The model under review builds one solid part; all positions refer to its coordinate system, in mm. Face numbers are marked on the shaded views. A direction names the side the tool comes from. Coordinates: 2 decimals unless noted, no trailing zeros. Write each loop counter-clockwise with the first axis right and the second up, starting at its lowest first coordinate (ties: lowest second). Pieces come first, ordered by that corner, then holes. Notation, with made-up numbers: (75, 86.25) - (85, 86.25) arc R29 cw to (85, 125.25) - close; hole circle Ø6 at (-25, 50). An arc over 180 degrees is marked (long way). Put each result on its own line as item: value.
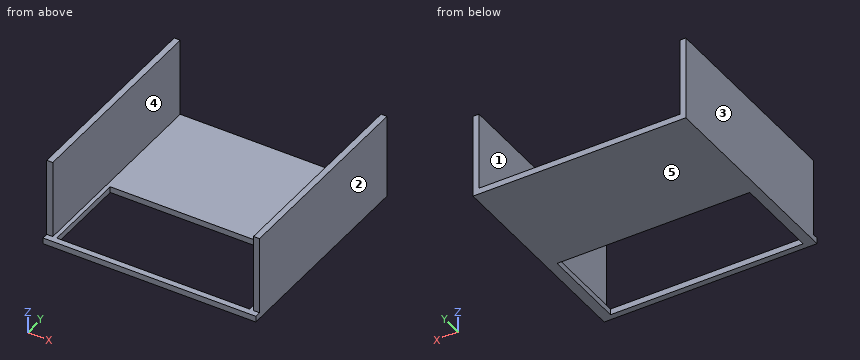
from build123d import *

# Parameters (mm, degrees)
SKETCH1_W                = 100
SKETCH1_H                = 77.5
BOSS_EXTRUDE1_DEPTH      = 3
BOSS_EXTRUDE2_DEPTH      = 102.5
BOSS_EXTRUDE2_DEPTH_BACK = 3
SKETCH2_W                = 106
SKETCH2_H                = 83.5
SKETCH2_W_2              = 100
SKETCH2_H_2              = 77.5
SKETCH3_W                = 106
SKETCH3_H                = 105.5
CUT_EXTRUDE1_DEPTH       = 41.5
CUT_EXTRUDE3_REACH       = 127.313
SKETCH6_W                = 96
SKETCH6_H                = 43
SKETCH7_W                = 106
SKETCH7_H                = 3
CUT_EXTRUDE4_DEPTH       = 39


with BuildPart() as part:
    # Sketch1 → Boss-Extrude1 (new body)
    with BuildSketch(Plane(origin=(0, 0, 0), x_dir=(1, 0, 0), z_dir=(0, 1, 0))):
        Rectangle(SKETCH1_W, SKETCH1_H)
    extrude(amount=BOSS_EXTRUDE1_DEPTH)

    # Sketch2 → Boss-Extrude2 (add, two sides: drawn at the far end of the back side and taken through both)
    with BuildSketch(Plane(origin=(0, 3, 0), x_dir=(1, 0, 0), z_dir=(0, 1, 0)).offset(-BOSS_EXTRUDE2_DEPTH_BACK)):
        Rectangle(SKETCH2_W, SKETCH2_H)
        Rectangle(SKETCH2_W_2, SKETCH2_H_2, mode=Mode.SUBTRACT)
    extrude(amount=BOSS_EXTRUDE2_DEPTH + BOSS_EXTRUDE2_DEPTH_BACK)

    # Sketch3 → Cut-Extrude1 (cut)
    with BuildSketch(Plane(origin=(0, 0, 41.75), x_dir=(-1, 0, 0), z_dir=(0, 0, -1))):
        with Locations((0, 52.75)):
            Rectangle(SKETCH3_W, SKETCH3_H)
    extrude(amount=CUT_EXTRUDE1_DEPTH, mode=Mode.SUBTRACT)

    # Sketch6 → Cut-Extrude3 (cut, up to next)
    with BuildSketch(Plane(origin=(0, 0, -41.75), x_dir=(-1, 0, 0), z_dir=(0, 0, -1)), mode=Mode.PRIVATE) as cut_extrude3_sk1:
        with Locations((0, 24.5)):
            Rectangle(SKETCH6_W, SKETCH6_H)
    cut_extrude3_tool1 = extrude(cut_extrude3_sk1.sketch, amount=-CUT_EXTRUDE3_REACH, mode=Mode.PRIVATE) & part.part
    add(cut_extrude3_tool1.solids().sort_by_distance((0, 24.5, -41.75))[0], mode=Mode.SUBTRACT)

    # Sketch7 → Cut-Extrude4 (cut)
    with BuildSketch(Plane.XY.offset(0.25)):
        with Locations((0, 1.5)):
            Rectangle(SKETCH7_W, SKETCH7_H)
    extrude(amount=-CUT_EXTRUDE4_DEPTH, mode=Mode.SUBTRACT)


solid = part.part
1. Consider section D-D on y = 68. State the section outline as (x, z) points, plus the area to 3 significant figures.
Determined:
outline: (-53, -41.75) - (53, -41.75) - (53, 0.25) - (50, 0.25) - (50, -38.75) - (-50, -38.75) - (-50, 0.25) - (-53, 0.25) - close
area: 552 mm^2
2. Consider section A-A on x = 44. State the section outline as (y, z) points, plus the area to 4 significant figures.
Determined:
outline: (0, -41.75) - (3, -41.75) - (3, -38.75) - (0, -38.75) - close; (46, -41.75) - (105.5, -41.75) - (105.5, -38.75) - (46, -38.75) - close
area: 187.5 mm^2
3. Consider section C-C on y = 15. State the section outline as (x, z) points, plus the area to 3 significant figures.
Determined:
outline: (-53, -41.75) - (-48, -41.75) - (-48, -38.75) - (-50, -38.75) - (-50, 0.25) - (-53, 0.25) - close; (48, -41.75) - (53, -41.75) - (53, 0.25) - (50, 0.25) - (50, -38.75) - (48, -38.75) - close
area: 264 mm^2
4. To check wall thickness, follow probe 1 along X at (y, z) = (66, -23); probe 2 along Y at (x, z) = (9, -39.5); probe 3 along X at (y, z) = (40.5, -40). State the ranges of each line that lie inside material, in increasing order.
Determined:
probe 1: x = -53 to -50, 50 to 53
probe 2: y = 0 to 3, 46 to 105.5
probe 3: x = -53 to -48, 48 to 53
5. Machinability: for the marked faces 4 and 5, which of the approach directions +Z, -Z, +X, -X, +Y, -Y give a long, thin tool a straight path to every point of the face, cutting with its end or side? Answer none if there is none.
Determined:
face 4: +Z, +Y, -Y
face 5: -Z, +X, -X, +Y, -Y
6. The part is to be moulded in two halves that separate along X. For the marked faces 1, 2 and 3, say which applies: +X half, -X half, draft (parallel to the pull), parting line (faces both ways), or undercut.
Determined:
face 1: undercut
face 2: +X half
face 3: -X half
7. Consider section B-B on z = -21.5. State the section outline as (x, y) points, plus the area to 3 significant figures.
Determined:
outline: (-53, 3) - (-50, 3) - (-50, 105.5) - (-53, 105.5) - close; (50, 3) - (53, 3) - (53, 105.5) - (50, 105.5) - close
area: 615 mm^2
8. For pin 1 Ø1 at (x, y) = (21, 59.5) entering from +Z; pin 2 Ø2.5 at (x, z) = (51, -14.5) entering from -Y, all flat-tipped, find the tip position at first contact; note any pin that passes through.
Determined:
pin 1: stops at z = -38.75
pin 2: stops at y = 3
